```python
from build123d import *

# Parameters (mm, degrees)
SKETCH_R        = 1
PAD_DEPTH       = 1.5
PAD001_DEPTH    = 16
SKETCH002_R     = 1.6
POCKET_DEPTH    = 40
POCKET001_DEPTH = 14.5
SKETCH006_W     = 5
SKETCH006_H     = 20
POCKET002_DEPTH = 20


with BuildPart() as part:
    # Sketch → Pad (new body)
    with BuildSketch(Plane.XY):
        with BuildLine():
            Line((9, 10.5), (30, 10.5))
            ThreePointArc((30, 10.5), (32, 8.5), (34, 10.5))
            Line((34, 10.5), (34, 14))
            ThreePointArc((34, 14), (-0.033107, 19.414422), (-34, 13.599057))
            Line((-34, 10.5), (-34, 13.599057))
            ThreePointArc((-34, 10.5), (-32, 8.5), (-30, 10.5))
            Line((-9, 10.5), (-30, 10.5))
            ThreePointArc((-9, 10.5), (-7, 8.5), (-5, 10.5))
            Line((-5, 10.5), (-5, -10.5))
            ThreePointArc((-5, -10.5), (-7, -8.5), (-9, -10.5))
            Line((-9, -10.5), (-30, -10.5))
            ThreePointArc((-30, -10.5), (-32, -8.5), (-34, -10.5))
            Line((-34, -10.5), (-34, -14.274102))
            ThreePointArc((-34, -14.274102), (0.024236, -20.149507), (34, -14))
            Line((34, -10.5), (34, -14))
            ThreePointArc((34, -10.5), (32, -8.5), (30, -10.5))
            Line((9, -10.5), (30, -10.5))
            ThreePointArc((9, -10.5), (7, -8.5), (5, -10.5))
            Line((5, 10.5), (5, -10.5))
            ThreePointArc((5, 10.5), (7, 8.5), (9, 10.5))
        make_face()
        with Locations((7, 10.5)):
            Circle(SKETCH_R, mode=Mode.SUBTRACT)
        with Locations((7, -10.5)):
            Circle(SKETCH_R, mode=Mode.SUBTRACT)
        with Locations((32, 10.5)):
            Circle(SKETCH_R, mode=Mode.SUBTRACT)
        with Locations((32, -10.5)):
            Circle(SKETCH_R, mode=Mode.SUBTRACT)
        with Locations((-7, 10.5)):
            Circle(SKETCH_R, mode=Mode.SUBTRACT)
        with Locations((-7, -10.5)):
            Circle(SKETCH_R, mode=Mode.SUBTRACT)
        with Locations((-32, 10.5)):
            Circle(SKETCH_R, mode=Mode.SUBTRACT)
        with Locations((-32, -10.5)):
            Circle(SKETCH_R, mode=Mode.SUBTRACT)
    extrude(amount=PAD_DEPTH)

    # Sketch001 → Pad001 (new body)
    with BuildSketch(Plane.XY.offset(1.5)):
        with BuildLine():
            Line((-34, 12.35), (-5, 12.35))
            Line((-5, 12.35), (-5, 10.5))
            Line((-5, 10.5), (-5, -10.5))
            Line((-5, -10.5), (-5, -12.35))
            Line((-34, -12.35), (-5, -12.35))
            Line((-34, -12.35), (-34, -14.265938))
            ThreePointArc((-34, -14.265938), (0.023508, -20.143886), (34, -14))
            Line((34, -12.35), (34, -14))
            Line((34, -12.35), (5, -12.35))
            Line((5, -10.5), (5, -12.35))
            Line((5, 10.5), (5, -10.5))
            Line((5, 12.35), (5, 10.5))
            Line((34, 12.35), (5, 12.35))
            Line((34, 12.35), (34, 14))
            ThreePointArc((34, 14), (-0.033512, 19.410124), (-34, 13.594018))
            Line((-34, 13.594018), (-34, 12.35))
        make_face()
    extrude(amount=PAD001_DEPTH)

    # Sketch002 → Pocket (cut)
    with BuildSketch(Plane(origin=(0, 0, 0), x_dir=(1, 0, 0), z_dir=(0, 0, -1))):
        with Locations((0, 15)):
            Circle(SKETCH002_R)
        with Locations((0, -15)):
            Circle(SKETCH002_R)
    extrude(amount=-POCKET_DEPTH, mode=Mode.SUBTRACT)

    # Sketch005 → Pocket001 (cut)
    with BuildSketch(Plane(origin=(0, 0, 0), x_dir=(1, 0, 0), z_dir=(0, 0, -1))):
        Polygon((1.680935, 12.27705), (3.198611, 15.094258), (1.517676, 17.817208), (-1.680935, 17.72295), (-3.198611, 14.905742), (-1.517676, 12.182792), align=None)
        Polygon((1.642986, -17.746015), (3.199612, -14.95014), (1.556626, -12.204125), (-1.642986, -12.253985), (-3.199612, -15.04986), (-1.556626, -17.795875), align=None)
    extrude(amount=-POCKET001_DEPTH, mode=Mode.SUBTRACT)

    # Sketch006 → Pocket002 (cut)
    with BuildSketch(Plane.XY.offset(17.5)):
        Rectangle(SKETCH006_W, SKETCH006_H)
    extrude(amount=-POCKET002_DEPTH, mode=Mode.SUBTRACT)


solid = part.part
```
Geometry check sheet. Reference: the model listing, model coordinates, mm. A direction names the side the tool comes from. Round coordinates to 2 decimals unless told otherwise and drop trailing zeros. Loops run counter-clockwise (first coordinate to the right, second up) from the corner with the lowest first, then second, coordinate; pieces in that order, holes last. Notation, with made-up numbers: M 89.25,43.5 L 125.25,43.5 A20 ccw 125.25,57.5 Z; hole C 63.25,33.25 d6. An arc over 180 degrees is marked long. Return JSON: item names as keys, results as strings. Group by question number.
(1) Go/stop test with flat-tipped pins: pin 1 (5 mm diameter, centred on x = 0.5, z = 5.5, fed in from -Y); pin 2 (5 mm diameter, centred on x = 10, z = 9, fed in from -Y); pin 3 (6 mm diameter, centred on x = 24, y = -8, fed in from +Z). Record where each tip stops, or that it passes through.
(2) Mould release check, pull along X, two halves, no side actions. Record for faces 3 (the face through (-7, -8.5, 0.7)), 4 (the face through (-3, 3, 17.5)): pulls with the +X half, pulls with the -X half, needs draft (parallel to the pull), parting line crosses it, or undercut.
(3) Set-up check for faces 1 (the face through (2.5, 0, 9)), 2 (the face through (2.39, 13.6, 7.15)): record each of +Z, -Z, +X, -X, +Y, -Y from which the full face is reachable in a straight line by a thin tool's end or side.
(4) Section check A-A, the plane y = -2. Enter the section's corners in (x, z), and give its area (3 significant figures).
(5) Section check B-B, the plane x = 0. Give the number of separate pieces and of enclosed holes in the cut face, and give its area (3 significant figures).
(6) Section check C-C, the plane z = 10.5. Enter the section's corners in (x, y).
(7) Scan lines: line 1 along X through (y, z) = (4, 15.5); line 2 along Y through (x, z) = (32, 1.2); line 3 along Y through (x, z) = (-16, 13). Record each from-to range of solid material in increasing order. Write a range as [from, to].
Data:
{
 "1": {"pin 1": "y = -20.14", "pin 2": "y = -19.83", "pin 3": "z = 1.5"},
 "2": {"face 3": "undercut", "face 4": "needs draft"},
 "3": {"face 1": "+Z, -Z", "face 2": "-Z"},
 "4": {"outline": "M -5,0 L -2.5,0 L -2.5,17.5 L -5,17.5 Z; M 2.5,0 L 5,0 L 5,17.5 L 2.5,17.5 Z", "area": "87.5 mm²"},
 "5": {"separate pieces": "4", "enclosed holes": "0", "area": "162 mm²"},
 "6": {"outline": "M -34,-14.27 A99.16 ccw 34,-14 L 34,-12.35 L 5,-12.35 L 5,12.35 L 34,12.35 L 34,14 A105.78 ccw -34,13.59 L -34,12.35 L -5,12.35 L -5,-12.35 L -34,-12.35 Z; hole M -3.2,-14.91 L -1.68,-17.72 L 1.52,-17.82 L 3.2,-15.09 L 1.68,-12.28 L -1.52,-12.18 Z; hole M -3.2,15.05 L -1.64,12.25 L 1.56,12.2 L 3.2,14.95 L 1.64,17.75 L -1.56,17.8 Z; hole M -2.5,-10 L 2.5,-10 L 2.5,10 L -2.5,10 Z"},
 "7": {"line 1": "[-5, -2.5], [2.5, 5]", "line 2": "[-14.72, -11.5], [-9.5, -8.5], [8.5, 9.5], [11.5, 14.64]", "line 3": "[-18.9, -12.35], [12.35, 18.1]"}
}
